```python
from build123d import *

# Parameters (mm, degrees)
F1_DEPTH = 25.4
F2_R     = 11.0288087202
F3_DEPTH = 25.4
F4_W     = 9.8473913968
F4_H     = 10.6680002064
F6_DEPTH = 50.8
F5_W     = 10.4628503323
F5_H     = 40.4153093696
F7_DEPTH = 76.2


with BuildPart() as f1:
    # F0 (on Top) → F1 (new body)
    with BuildSketch(Plane.XY):
        with BuildLine():
            Line((-44.45, -25.4), (44.45, -25.4))
            Line((44.45, -25.4), (44.45, 25.4))
            Line((44.45, 25.4), (-44.45, 25.4))
            Line((-44.45, 25.4), (-44.45, 25.0481939564))
            ThreePointArc((-44.45, 25.0481939564), (-26.738252197, 17.711747803), (-19.4018060436, 0))
            ThreePointArc((-19.4018060436, 0), (-26.738252197, -17.711747803), (-44.45, -25.0481939564))
            Line((-44.45, -25.0481939564), (-44.45, -25.4))
        make_face()
        with BuildLine():
            ThreePointArc((-44.45, 25.0481939564), (-69.4981939564, 0), (-44.45, -25.0481939564))
            Line((-44.45, -25.0481939564), (-44.45, 25.0481939564))
        make_face()
        with BuildLine():
            Line((-44.45, 25.0481939564), (-44.45, -25.0481939564))
            ThreePointArc((-44.45, -25.0481939564), (-26.738252197, -17.711747803), (-19.4018060436, 0))
            ThreePointArc((-19.4018060436, 0), (-26.738252197, 17.711747803), (-44.45, 25.0481939564))
        make_face()
    extrude(amount=F1_DEPTH)

    # F2 (on Top) → F3 (cut)
    with BuildSketch(Plane.XY):
        with Locations((-50.4678487778, 0)):
            Circle(F2_R)
    extrude(amount=F3_DEPTH, mode=Mode.SUBTRACT)

    # F4 (on Top) → F6 (join)
    with BuildSketch(Plane.XY):
        with Locations((39.5263043016, 20.0659998968)):
            Rectangle(F4_W, F4_H)
    extrude(amount=F6_DEPTH)

    # F5 (on Top) → F7 (join)
    with BuildSketch(Plane.XY):
        with Locations((39.2185748339, -5.4365769029)):
            Rectangle(F5_W, F5_H)
    extrude(amount=F7_DEPTH)


solid = f1.part
```
Work out the finished part from the listing and answer in its coordinate system (mm). A direction names the side the tool comes from. Round coordinates to 2 decimals unless told otherwise and drop trailing zeros. Write each loop counter-clockwise with the first axis right and the second up, starting at its lowest first coordinate (ties: lowest second). Pieces come first, ordered by that corner, then holes. Notation, with made-up numbers: (58.5, 57) - (77.5, 57) arc R29 ccw to (77.5, 96) - close; hole circle Ø5 at (78.5, 24). An arc over 180 degrees is marked (long way). Return JSON: item names as keys, results as strings. Group by question number.
Q1. The mould has two halves that part along Y. Classify faces 4 (the cylindrical face through (-40.28, -4.22, 12.52)), 5 (the flat face through (-6, -25.4, 13)), 6 (the flat face through (44.45, 0, 38)), 7 (the flat face through (1, 25.4, 14)): released by +Y, released by -Y, zero draft, split by the parting line, or undercut.
Q2. The part is cut by section C-C on z = 13. Write down the section's boundary in (x, y), then the cut area to 3 significant figures.
Q3. The part is cut by section D-D on x = 20. Write down the section's boundary in (y, z), then the cut area to 3 significant figures.
Q4. The part is cut by section B-B on x = -53.5. Write down the section's boundary in (y, z).
Q5. Each of these flat-tipped pins is pushed along its axis until it touches: pin 1 Ø3 at (x, y) = (37, 19.5) entering from +Z; pin 2 Ø20.5 at (x, z) = (-9.5, 8.5) entering from -Y; pin 3 Ø20 at (y, z) = (1.5, 43) entering from -X. Where does it stop, or does it pass through?
Q6. For faces 1 (the flat face through (39, 20, 50.8)), 2 (the flat face through (39, -25.644, 38)), 3 (the flat face through (34.603, 20, 38)), determine the directions among +Z, -Z, +X, -X, +Y, -Y from which every point of the face is accessible in a straight line to the end or side of a thin tool.
Q7. Find the intervals of material crossed by L1, parallel to Z at x = 30.5, y = 14; L2, parallel to X at y = 9, z = 64.5; L3, parallel to X at y = -9, z = 22, in increasing order.
Q8. The part is cut by section A-A on y = 0. Write down the section's boundary in (x, z), then the cut area to 3 significant figures.
Solved:
{
 "1": {"face 4": "undercut", "face 5": "released by -Y", "face 6": "zero draft", "face 7": "released by +Y"},
 "2": {"outline": "(-44.45, -25.4) - (33.99, -25.4) - (33.99, -25.64) - (44.45, -25.64) - (44.45, 25.4) - (-44.45, 25.4) - (-44.45, 25.05) arc R25.05 ccw to (-44.45, -25.05) - close; hole circle Ø22.06 at (-50.47, 0)", "area": "5,120 mm²"},
 "3": {"outline": "(-25.4, 0) - (25.4, 0) - (25.4, 25.4) - (-25.4, 25.4) - close", "area": "1,290 mm²"},
 "4": {"outline": "(-23.36, 0) - (-10.6, 0) - (-10.6, 25.4) - (-23.36, 25.4) - close; (10.6, 0) - (23.36, 0) - (23.36, 25.4) - (10.6, 25.4) - close"},
 "5": {"pin 1": "z = 50.8", "pin 2": "y = -25.4", "pin 3": "x = 33.99"},
 "6": {"face 1": "+Z, +X, -X, +Y", "face 2": "+Z, -Z, +X, -X, -Y", "face 3": "+Z, -X, +Y"},
 "7": {"L1": "0 to 25.4", "L2": "33.99 to 44.45", "L3": "-67.83 to -56.84, -44.09 to 44.45"},
 "8": {"outline": "(-69.5, 0) - (-61.5, 0) - (-61.5, 25.4) - (-69.5, 25.4) - close; (-39.44, 0) - (44.45, 0) - (44.45, 76.2) - (33.99, 76.2) - (33.99, 25.4) - (-39.44, 25.4) - close", "area": "2,870 mm²"}
}
